from build123d import *

# Parameters (mm, degrees)
SKETCH1_R               = 1.6
SKETCH1_R_2             = 5.7
BOSS_EXTRUDE1_DEPTH     = 16
SKETCH2_R               = 1.6
CUT_EXTRUDE1_DEPTH      = 18.4
SKETCH3_W               = 8
SKETCH3_H               = 4
CUT_EXTRUDE2_DEPTH      = 14.9
SKETCH4_R               = 2.6
CUT_EXTRUDE3_DEPTH      = 25
SKETCH5_R               = 6
CUT_EXTRUDE4_DEPTH      = 6
SKETCH6_R               = 4.025
CUT_EXTRUDE5_DEPTH      = 17.4
SKETCH7_R               = 7.95
CUT_EXTRUDE6_DEPTH      = 11
SKETCH8_R               = 7.95
CUT_EXTRUDE7_DEPTH      = 11
BOSS_EXTRUDE2_DEPTH     = 7.7
SKETCH10_R              = 1.6
CUT_EXTRUDE8_DEPTH      = 21
CUT_EXTRUDE9_DEPTH      = 20
CUT_EXTRUDE9_DEPTH_BACK = 20
FILLET2_R               = 0.5


with BuildPart() as part:
    # Sketch1 → Boss-Extrude1 (new body, symmetric)
    with BuildSketch(Plane.XY):
        with BuildLine():
            Line((0, 0), (23, 0))
            Line((23, 0), (23, 11.85))
            Line((23, 11.85), (40, 11.85))
            Line((40, 11.85), (40, 22.85))
            Line((40, 22.85), (24.3, 22.85))
            Line((24.3, 22.85), (24.3, 24.85))
            Line((24.3, 24.85), (40, 24.85))
            Line((40, 24.85), (40, 32.85))
            Line((40, 32.85), (15.939721203, 32.85))
            ThreePointArc((15.939721203, 32.85), (-0.817389789, 43.335843617), (1.211999203, 23.672800478))
            ThreePointArc((1.211999203, 23.672800478), (2.953099737, 18.191047558), (0, 13.255437353))
            Line((0, 13.255437353), (0, 0))
        make_face()
        with Locations((28.1, 28.85)):
            Circle(SKETCH1_R, mode=Mode.SUBTRACT)
        with Locations((28.1, 18.85)):
            Circle(SKETCH1_R, mode=Mode.SUBTRACT)
        with Locations((5, 34)):
            Circle(SKETCH1_R_2, mode=Mode.SUBTRACT)
    extrude(amount=BOSS_EXTRUDE1_DEPTH, both=True)

    # Sketch2 → Cut-Extrude1 (cut)
    with BuildSketch(Plane(origin=(0, 0, -16), x_dir=(-1, 0, 0), z_dir=(0, 0, -1))):
        with BuildLine():
            Line((-23, 0), (-15, 0))
            Line((-15, 0), (-15, 16.5))
            Line((-15, 16.5), (-2.538348415, 16.5))
            ThreePointArc((-2.538348415, 16.5), (-2.706537293, 16.994418404), (-2.837397166, 17.5))
            Line((-2.837397166, 17.5), (-15, 17.5))
            Line((-15, 17.5), (-15, 29.417424305))
            ThreePointArc((-15, 29.417424305), (-15.609600605, 31.095456144), (-15.939721203, 32.85))
            Line((-15.939721203, 32.85), (-40, 32.85))
            Line((-40, 32.85), (-40, 24.85))
            Line((-40, 24.85), (-24.3, 24.85))
            Line((-24.3, 24.85), (-24.3, 22.85))
            Line((-24.3, 22.85), (-40, 22.85))
            Line((-40, 22.85), (-40, 11.85))
            Line((-40, 11.85), (-23, 11.85))
            Line((-23, 11.85), (-23, 0))
        make_face()
        with Locations((-28.1, 18.85)):
            Circle(SKETCH2_R, mode=Mode.SUBTRACT)
        with Locations((-28.1, 28.85)):
            Circle(SKETCH2_R, mode=Mode.SUBTRACT)
    extrude(amount=-CUT_EXTRUDE1_DEPTH, mode=Mode.SUBTRACT)

    # Sketch3 → Cut-Extrude2 (cut)
    with BuildSketch(Plane(origin=(0, 0, -16), x_dir=(-1, 0, 0), z_dir=(0, 0, -1))):
        with Locations((-8.7, 21.5)):
            Rectangle(SKETCH3_W, SKETCH3_H)
    extrude(amount=-CUT_EXTRUDE2_DEPTH, mode=Mode.SUBTRACT)

    # Sketch4 → Cut-Extrude3 (cut)
    with BuildSketch(Plane.XZ):
        with Locations((8.7, -7.6)):
            Circle(SKETCH4_R)
    extrude(amount=-CUT_EXTRUDE3_DEPTH, mode=Mode.SUBTRACT)

    # Sketch5 → Cut-Extrude4 (cut)
    with BuildSketch(Plane.XZ):
        with Locations((8.7, -7.6)):
            Circle(SKETCH5_R)
    extrude(amount=-CUT_EXTRUDE4_DEPTH, mode=Mode.SUBTRACT)

    # Sketch6 → Cut-Extrude5 (cut)
    with BuildSketch(Plane.ZY):
        with Locations((4.2, 17)):
            Circle(SKETCH6_R)
    extrude(amount=-CUT_EXTRUDE5_DEPTH, mode=Mode.SUBTRACT)

    # Sketch7 → Cut-Extrude6 (cut)
    with BuildSketch(Plane(origin=(0, 0, -16), x_dir=(-1, 0, 0), z_dir=(0, 0, -1))):
        with Locations((-5, 34)):
            Circle(SKETCH7_R)
    extrude(amount=-CUT_EXTRUDE6_DEPTH, mode=Mode.SUBTRACT)

    # Sketch8 → Cut-Extrude7 (cut)
    with BuildSketch(Plane.XY.offset(16)):
        with Locations((5, 34)):
            Circle(SKETCH8_R)
    extrude(amount=-CUT_EXTRUDE7_DEPTH, mode=Mode.SUBTRACT)

    # Sketch9 → Boss-Extrude2 (add)
    with BuildSketch(Plane(origin=(24.3, 0, 0), x_dir=(0, 0, -1), z_dir=(1, 0, 0))):
        Polygon((-15.7, 22.85), (-14.7, 22.85), (-14.8, 23.85), (-15.6, 23.85), align=None)
        Polygon((-13.6, 23.85), (-13.7, 22.85), (-12.7, 22.85), (-12.8, 23.85), align=None)
        Polygon((-11.6, 23.85), (-11.7, 22.85), (-10.7, 22.85), (-10.8, 23.85), align=None)
        Polygon((-9.6, 23.85), (-9.7, 22.85), (-8.7, 22.85), (-8.8, 23.85), align=None)
        Polygon((-7.6, 23.85), (-7.7, 22.85), (-6.7, 22.85), (-6.8, 23.85), align=None)
        Polygon((-5.6, 23.85), (-5.7, 22.85), (-4.7, 22.85), (-4.8, 23.85), align=None)
        Polygon((-3.6, 23.85), (-3.7, 22.85), (-2.7, 22.85), (-2.8, 23.85), align=None)
    extrude(amount=BOSS_EXTRUDE2_DEPTH)

    # Sketch10 → Cut-Extrude8 (cut)
    with BuildSketch(Plane(origin=(0, 32.85, 0), x_dir=(1, 0, 0), z_dir=(0, 1, 0))):
        with Locations((36, -9.2)):
            Circle(SKETCH10_R)
    extrude(amount=-CUT_EXTRUDE8_DEPTH, mode=Mode.SUBTRACT)

    # Sketch11 → Cut-Extrude9 (cut, two sides)
    with BuildSketch(Plane(origin=(0, 0, 2.4), x_dir=(-1, 0, 0), z_dir=(0, 0, -1))) as cut_extrude9_sk:
        Polygon((-23, 11.85), (-17.4, 11.85), (-17.4, 32.85), (-17.4, 56.269186849), (20.068849224, 56.269186849), (20.068849224, -12.231640917), (-23, -11.328049524), (-29.029830536, 8.113428838), align=None)
    extrude(amount=CUT_EXTRUDE9_DEPTH, mode=Mode.SUBTRACT)
    extrude(cut_extrude9_sk.sketch, amount=-CUT_EXTRUDE9_DEPTH_BACK, mode=Mode.SUBTRACT)

    # Fillet2
    fillet2_edges = [part.edges().sort_by_distance(p)[0] for p in [
        (28.7, 11.85, 16),
        (17.4, 22.35, 2.4),
        (40, 17.35, 16),
        (40, 32.85, 9.2),
        (40, 24.85, 9.2),
        (40, 22.85, 9.2),
        (40, 11.85, 9.2),
        (28.7, 32.85, 2.4),
        (17.4, 32.85, 9.2),
        (17.4, 22.35, 16),
        (17.4, 11.85, 9.2),
        (40, 28.85, 16),
        (28.7, 32.85, 16),
        (28.7, 11.85, 2.4),
        (40, 17.35, 2.4),
        (40, 28.85, 2.4),
    ]]
    fillet(fillet2_edges, radius=FILLET2_R)


solid = part.part
For this review, take the finished solid that the model builds, in its own axes (mm). A direction names the side the tool comes from. Coordinates: 2 decimals unless noted, no trailing zeros. Loops run counter-clockwise (first coordinate to the right, second up) from the corner with the lowest first, then second, coordinate; pieces in that order, holes last. Notation, with made-up numbers: (16.25, 54.25) - (27.25, 54.25) arc R21 ccw to (27.25, 74.25) - close; hole circle Ø6 at (-14.5, 3). An arc over 180 degrees is marked (long way). Return JSON: item names as keys, results as strings.
Item 1: Take a section at B-B (x = 36). Give the boundary of the cut face in (y, z), then the cut area to 3 significant figures.
Determined:
{"outline": "(11.85, 2.9) arc R0.5 ccw to (12.35, 2.4) - (22.85, 2.4) - (22.85, 7.6) - (11.85, 7.6) - close; (11.85, 10.8) - (22.85, 10.8) - (22.85, 16) - (12.35, 16) arc R0.5 ccw to (11.85, 15.5) - close; (24.85, 2.4) - (32.35, 2.4) arc R0.5 ccw to (32.85, 2.9) - (32.85, 7.6) - (24.85, 7.6) - close; (24.85, 10.8) - (32.85, 10.8) - (32.85, 15.5) arc R0.5 ccw to (32.35, 16) - (24.85, 16) - close", "area": "197 mm2"}
Item 2: Take a section at D-D (y = 19.5). Give the boundary of the cut face in (x, z).
Determined:
{"outline": "(17.4, 2.9) arc R0.5 ccw to (17.9, 2.4) - (26.64, 2.4) - (26.64, 16) - (17.9, 16) arc R0.5 ccw to (17.4, 15.5) - close; (29.56, 2.4) - (39.5, 2.4) arc R0.5 ccw to (40, 2.9) - (40, 15.5) arc R0.5 ccw to (39.5, 16) - (29.56, 16) - close; hole circle Ø3.2 at (36, 9.2)"}
Item 3: Mouldability with a two-part tool opening along Z and no side actions: class faces 1 (the flat face through (29, 11.85, 9)), 2 (the flat face through (28.1, 23.34, 10.75)), 3 (the flat face through (28.1, 23.36, 13.65)), 4 (the flat face through (28.1, 23.34, 2.75)) as pulls with the +Z half, pulls with the -Z half, needs draft (parallel to the pull), parting line crosses it, or undercut.
Determined:
{"face 1": "needs draft", "face 2": "undercut", "face 3": "undercut", "face 4": "pulls with the -Z half"}
Item 4: Insertion check: pin 1 (1.1 mm diameter, centred on y = 23, z = 13, fed in from +X); pin 2 (2.5 mm diameter, centred on x = 36, z = 9.2, fed in from +Y); pin 3 (1.1 mm diameter, centred on y = 23.5, z = 3, fed in from +X). Each pin has a flat end and moves straight along its axis. Give the tip position at first contact, or say it passes through.
Determined:
{"pin 1": "stops at x = 39.99", "pin 2": "passes through", "pin 3": "stops at x = 32"}
Item 5: For line 1 (Y direction, x = 28.1, z = 7.25); line 2 (Y direction, x = 33.75, z = 8), list the stretches that pass through material, from the lowest coordinate up.
Determined:
{"line 1": "y = 11.85 to 17.25, 20.45 to 23.85, 24.85 to 27.25, 30.45 to 32.85", "line 2": "y = 11.85 to 22.85, 24.85 to 32.85"}
Item 6: For faces 5 (the flat face through (28.1, 23.34, 6.75)), 6 (the flat face through (28.1, 23.36, 15.65)), 7 (the flat face through (17.4, 22, 9)), 8 (the flat face through (32, 23.4, 5.2)), 9 (the cylindrical face through (26.83, 17.88, 9.1)), list the 3-axis set-ups (+Z, -Z, +X, -X, +Y, -Y) from which the entire face can be reached by the end or side of a thin tool; tool diameter is ignored.
Determined:
{"face 5": "+X", "face 6": "+Z, +X", "face 7": "+Z, -Z, -X, +Y, -Y", "face 8": "+Z, -Z, +X", "face 9": "+Z, -Z"}
Item 7: Take a section at C-C (z = 14). Give the boundary of the cut face in (x, y), then the cut area to 3 significant figures.
Determined:
{"outline": "(17.4, 12.35) arc R0.5 ccw to (17.9, 11.85) - (39.5, 11.85) arc R0.5 ccw to (40, 12.35) - (40, 22.35) arc R0.5 ccw to (39.5, 22.85) - (24.3, 22.85) - (24.3, 24.85) - (39.5, 24.85) arc R0.5 ccw to (40, 25.35) - (40, 32.35) arc R0.5 ccw to (39.5, 32.85) - (17.9, 32.85) arc R0.5 ccw to (17.4, 32.35) - close; hole circle Ø3.2 at (28.1, 18.85); hole circle Ø3.2 at (28.1, 28.85)", "area": "427 mm2"}
Item 8: Take a section at A-A (y = 28.85). Give the boundary of the cut face in (x, z), then the cut area to 3 significant figures.
Determined:
{"outline": "(17.4, 2.9) arc R0.5 ccw to (17.9, 2.4) - (26.5, 2.4) - (26.5, 16) - (17.9, 16) arc R0.5 ccw to (17.4, 15.5) - close; (29.7, 2.4) - (39.5, 2.4) arc R0.5 ccw to (40, 2.9) - (40, 15.5) arc R0.5 ccw to (39.5, 16) - (29.7, 16) - close; hole circle Ø3.2 at (36, 9.2)", "area": "256 mm2"}
